from build123d import *

# Parameters (mm, degrees)
F0_R      = 2.2
F0_R_2    = 1.7
F1_DEPTH  = 46
F3_DEPTH  = 3
F5_R      = 1.7
F6_DEPTH  = 78.501
F8_DEPTH  = 2
F10_DEPTH = 2
F12_DEPTH = 2
F13_R     = 16
F14_DEPTH = 5
F15_D     = 3.4


with BuildPart() as f1:
    # F0 (on Top) → F1 (new body)
    with BuildSketch(Plane.XY):
        with BuildLine():
            ThreePointArc((-31, -14.7792156109), (-30, -6.5), (-29, -14.7792156109))
            Line((-29, -14.7792156109), (-29, -22))
            Line((-29, -22), (-24, -22))
            Line((-24, -22), (-24, -5))
            Line((-24, -5), (0, -5))
            Line((0, -5), (0, 0))
            Line((0, 0), (-24, 0))
            ThreePointArc((-24, 0), (-24.9502475308, 3.2403703492), (-27.5, 5.4543560573))
            ThreePointArc((-27.5, 5.4543560573), (-30, 6), (-32.5, 5.4543560573))
            ThreePointArc((-32.5, 5.4543560573), (-35.0497524692, 3.2403703492), (-36, 0))
            Line((-36, 0), (-36, -22))
            Line((-36, -22), (-31, -22))
            Line((-31, -22), (-31, -14.7792156109))
        make_face()
        with Locations((-30, 1.5)):
            Circle(F0_R, mode=Mode.SUBTRACT)
        with BuildLine():
            Line((0, 0), (0, -5))
            Line((0, -5), (24, -5))
            Line((24, -5), (24, -22))
            Line((24, -22), (29, -22))
            Line((29, -22), (29, -14.7792156109))
            ThreePointArc((29, -14.7792156109), (30, -6.5), (31, -14.7792156109))
            Line((31, -14.7792156109), (31, -22))
            Line((31, -22), (36, -22))
            Line((36, -22), (36, 0))
            ThreePointArc((36, 0), (35.0497524692, 3.2403703492), (32.5, 5.4543560573))
            ThreePointArc((32.5, 5.4543560573), (30, 6), (27.5, 5.4543560573))
            ThreePointArc((27.5, 5.4543560573), (24.9502475308, 3.2403703492), (24, 0))
            Line((24, 0), (0, 0))
        make_face()
        with Locations((30, 1.5)):
            Circle(F0_R, mode=Mode.SUBTRACT)
        with BuildLine():
            Line((-32.5, 33.1698729811), (-32.5, 5.4543560573))
            ThreePointArc((-32.5, 5.4543560573), (-30, 6), (-27.5, 5.4543560573))
            Line((-27.5, 5.4543560573), (-27.5, 33.1698729811))
            ThreePointArc((-27.5, 33.1698729811), (-30, 32.5), (-32.5, 33.1698729811))
        make_face()
        with BuildLine():
            ThreePointArc((-25, 37.5), (-32.5, 41.8301270189), (-32.5, 33.1698729811))
            Line((-32.5, 33.1698729811), (-27.5, 33.1698729811))
            ThreePointArc((-27.5, 33.1698729811), (-25.6698729811, 35), (-25, 37.5))
        make_face()
        with Locations((-30, 37.5)):
            Circle(F0_R_2, mode=Mode.SUBTRACT)
        with BuildLine():
            Line((-27.5, 33.1698729811), (-32.5, 33.1698729811))
            ThreePointArc((-32.5, 33.1698729811), (-30, 32.5), (-27.5, 33.1698729811))
        make_face()
        with BuildLine():
            Line((27.5, 33.1698729811), (27.5, 5.4543560573))
            ThreePointArc((27.5, 5.4543560573), (30, 6), (32.5, 5.4543560573))
            Line((32.5, 5.4543560573), (32.5, 33.1698729811))
            ThreePointArc((32.5, 33.1698729811), (30, 32.5), (27.5, 33.1698729811))
        make_face()
        with BuildLine():
            ThreePointArc((35, 37.5), (27.5, 41.8301270189), (27.5, 33.1698729811))
            ThreePointArc((27.5, 33.1698729811), (30, 32.5), (32.5, 33.1698729811))
            ThreePointArc((32.5, 33.1698729811), (34.3301270189, 35), (35, 37.5))
        make_face()
        with Locations((30, 37.5)):
            Circle(F0_R_2, mode=Mode.SUBTRACT)
    extrude(amount=F1_DEPTH)

    # F2 (on face) → F3 (cut)
    with BuildSketch(Plane.XY.offset(46)):
        Polygon((-28.0536441704, -1.9095501636), (-26.0740650281, 1.4808185114), (-28.0204208576, 4.890368675), (-31.9463558296, 4.9095501636), (-33.9259349719, 1.5191814886), (-31.9795791424, -1.890368675), align=None)
        Polygon((33.9259349719, 1.5191814886), (31.9463558296, 4.9095501636), (28.0204208576, 4.890368675), (26.0740650281, 1.4808185114), (28.0536441704, -1.9095501636), (31.9795791424, -1.890368675), align=None)
    extrude(amount=-F3_DEPTH, mode=Mode.SUBTRACT)

    # F5 (on offset) → F6 (cut, through all)
    with BuildSketch(Plane(origin=(-42.5, 0, 0), x_dir=(0, -1, 0), z_dir=(-1, 0, 0))):
        Polygon((-43.1698729811, 46), (-43.1698729811, 8), (-33.1698729811, 8), (-5.4543560573, 46), align=None)
        with Locations((17, 39)):
            Circle(F5_R)
        with Locations((17, 23)):
            Circle(F5_R)
        with Locations((17, 7)):
            Circle(F5_R)
    extrude(amount=-F6_DEPTH, mode=Mode.SUBTRACT)

    # F7 (on face) → F8 (cut)
    with BuildSketch(Plane.XY.offset(8)):
        Polygon((-28.3256842194, 34.6), (-26.6513684387, 37.5), (-28.3256842194, 40.4), (-31.6743157806, 40.4), (-33.3486315613, 37.5), (-31.6743157806, 34.6), align=None)
        Polygon((28.3256842194, 40.4), (26.6513684387, 37.5), (28.3256842194, 34.6), (31.6743157806, 34.6), (33.3486315613, 37.5), (31.6743157806, 40.4), align=None)
    extrude(amount=-F8_DEPTH, mode=Mode.SUBTRACT)

    # F9 (on face) → F10 (cut)
    with BuildSketch(Plane(origin=(24, 0, 0), x_dir=(0, -1, 0), z_dir=(-1, 0, 0))):
        Polygon((15.3256842194, 36.1), (18.6743157806, 36.1), (20.3486315613, 39), (18.6743157806, 41.9), (15.3256842194, 41.9), (13.6513684387, 39), align=None)
        Polygon((15.3256842194, 20.1), (18.6743157806, 20.1), (20.3486315613, 23), (18.6743157806, 25.9), (15.3256842194, 25.9), (13.6513684387, 23), align=None)
        Polygon((15.3256842194, 4.1), (18.6743157806, 4.1), (20.3486315613, 7), (18.6743157806, 9.9), (15.3256842194, 9.9), (13.6513684387, 7), align=None)
    extrude(amount=-F10_DEPTH, mode=Mode.SUBTRACT)

    # F11 (on face) → F12 (cut)
    with BuildSketch(Plane.YZ.offset(-24)):
        Polygon((-18.6743157806, 36.1), (-15.3256842194, 36.1), (-13.6513684387, 39), (-15.3256842194, 41.9), (-18.6743157806, 41.9), (-20.3486315613, 39), align=None)
        Polygon((-18.6743157806, 20.1), (-15.3256842194, 20.1), (-13.6513684387, 23), (-15.3256842194, 25.9), (-18.6743157806, 25.9), (-20.3486315613, 23), align=None)
        Polygon((-18.6743157806, 4.1), (-15.3256842194, 4.1), (-13.6513684387, 7), (-15.3256842194, 9.9), (-18.6743157806, 9.9), (-20.3486315613, 7), align=None)
    extrude(amount=-F12_DEPTH, mode=Mode.SUBTRACT)

    # F13 (on face) → F14 (cut, through all)
    with BuildSketch(Plane(origin=(0, 0, 0), x_dir=(-1, 0, 0), z_dir=(0, 1, 0))):
        with Locations((0, 23)):
            Circle(F13_R)
    extrude(amount=-F14_DEPTH, mode=Mode.SUBTRACT)

    # F15 (through all)
    with Locations(Plane(origin=(0, 0, 0), x_dir=(-1, 0, 0), z_dir=(0, 1, 0))):
        with Locations((-15.5, 38.5), (15.5, 38.5), (15.5, 7.5), (-15.5, 7.5)):
            Hole(F15_D / 2)


solid = f1.part
Model file for the job. Use its own axes, mm. A direction names the side the tool comes from. Give positions to 0.01 mm unless a question says otherwise; leave off trailing zeros. Write each loop counter-clockwise with the first axis right and the second up, starting at its lowest first coordinate (ties: lowest second). Pieces come first, ordered by that corner, then holes. Notation, with made-up numbers: M -35.75,42.5 L -31.75,42.5 A24 cw -31.75,74.5 Z; hole C 4,-9 d4. An arc over 180 degrees is marked long. One line per item, written item: value. Start each with the question number.
Q1. Two-plate mould, pull along Z, no slides. Class faces 1 (the flat face through (30, 34.6, 7)), 2 (the flat face through (-24.986, -14.477, 24.43)): +Z half, -Z half, draft (parallel to the pull), parting line (faces both ways), or undercut.
Q2. Saw through at A-A, the plane y = -3.5. Write the cut outline in (x, z), plus the area to 3 significant figures.
Q3. Saw through at C-C, the plane z = 13. State how many separate pieces and enclosed holes the cut face has, plus the area to 3 significant figures.
Q4. Drop flat-ended pins along their axis: pin 1 Ø2 at (y, z) = (-17, 7) entering from -X; pin 2 Ø2 at (y, z) = (11, 10) entering from +X; pin 3 Ø4.5 at (x, y) = (31.5, 37) entering from +Z; pin 4 Ø8 at (x, z) = (-19.5, 21.5) entering from -Y. Give the stop position or say it passes through.
Q5. Saw through at D-D, the plane y = -10.7. Write the cut outline in (x, z), plus the area to 3 significant figures.
Q6. Probe probe 1 along Z at (x, y) = (28.1, -17); probe 2 along X at (y, z) = (-9.5, 19); probe 3 along X at (y, z) = (10.5, 13). List the from-to ranges inside material, lowest first. Write a range as [from, to].
Q7. 3-axis set-ups, long thin cutter, end or side, ignore diameter. For faces 3 (the flat face through (-24.99, -19.5, 24.47)), 4 (the flat face through (-27.5, 16, 18)), 5 (the flat face through (-27.034, 3.162, 44.521)): which of +Z, -Z, +X, -X, +Y, -Y reach the whole face in a straight line?
Q8. Saw through at B-B, the plane x = 0. Write the cut outline in (y, z).
Output values:
1. face 1: draft
1. face 2: undercut
2. outline: M -36,0 L 36,0 L 36,46 L -36,46 Z; hole C -15.5,7.5 d3.4; hole C -15.5,38.5 d3.4; hole C 0,23 d32; hole C 15.5,7.5 d3.4; hole C 15.5,38.5 d3.4
2. area: 2,470 mm²
3. separate pieces: 2
3. enclosed holes: 2
3. area: 823 mm²
4. pin 1: passes through
4. pin 2: stops at x = 32.5
4. pin 3: stops at z = 8
4. pin 4: stops at y = -5
5. outline: M -36,0 L -34.2,0 L -34.2,46 L -36,46 Z; M -25.8,0 L -24,0 L -24,46 L -25.8,46 Z; M 24,0 L 25.8,0 L 25.8,46 L 24,46 Z; M 34.2,0 L 36,0 L 36,46 L 34.2,46 Z
5. area: 331 mm²
6. probe 1: z = [0, 5.3], [8.7, 21.3], [24.7, 37.3], [40.7, 46]
6. probe 2: x = [-36, -34.02], [-25.98, -24], [24, 25.98], [34.02, 36]
6. probe 3: x = [-32.5, -27.5], [27.5, 32.5]
7. face 3: none
7. face 4: +Z, -Z
7. face 5: +Z
8. outline: M -5,0 L 0,0 L 0,7 L -5,7 Z; M -5,39 L 0,39 L 0,46 L -5,46 Z
